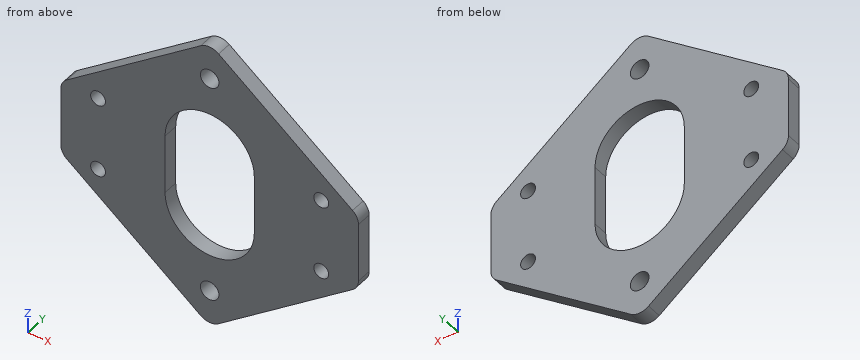
```python
from build123d import *

# Parameters (mm, degrees)
F0_R     = 12.7
F0_R_2   = 15.875
F1_DEPTH = 12.7


with BuildPart() as f1:
    # F0 (on Front) → F1 (new body, symmetric)
    with BuildSketch(Plane.XZ):
        with BuildLine():
            Line((254, -50.8), (254, 50.8))
            ThreePointArc((254, 50.8), (251.318451, 62.159225), (243.84, 71.12))
            Line((243.84, 71.12), (15.24, 242.57))
            ThreePointArc((15.24, 242.57), (0, 247.65), (-15.24, 242.57))
            Line((-15.24, 242.57), (-243.84, 71.12))
            ThreePointArc((-243.84, 71.12), (-251.318451, 62.159225), (-254, 50.8))
            Line((-254, 50.8), (-254, -50.8))
            ThreePointArc((-254, -50.8), (-251.318451, -62.159225), (-243.84, -71.12))
            Line((-243.84, -71.12), (-15.24, -242.57))
            ThreePointArc((-15.24, -242.57), (0, -247.65), (15.24, -242.57))
            Line((15.24, -242.57), (243.84, -71.12))
            ThreePointArc((243.84, -71.12), (251.318451, -62.159225), (254, -50.8))
        make_face()
        with Locations((-190.5, -63.5)):
            Circle(F0_R, mode=Mode.SUBTRACT)
        with Locations((0, -190.5)):
            Circle(F0_R_2, mode=Mode.SUBTRACT)
        with Locations((190.5, -63.5)):
            Circle(F0_R, mode=Mode.SUBTRACT)
        with Locations((-190.5, 63.5)):
            Circle(F0_R, mode=Mode.SUBTRACT)
        with BuildLine():
            ThreePointArc((-76.2, 50.8), (0, 127), (76.2, 50.8))
            Line((76.2, 50.8), (76.2, -50.8))
            ThreePointArc((76.2, -50.8), (0, -127), (-76.2, -50.8))
            Line((-76.2, -50.8), (-76.2, 50.8))
        make_face(mode=Mode.SUBTRACT)
        with Locations((190.5, 63.5)):
            Circle(F0_R, mode=Mode.SUBTRACT)
        with Locations((0, 190.5)):
            Circle(F0_R_2, mode=Mode.SUBTRACT)
    extrude(amount=F1_DEPTH, both=True)


solid = f1.part
```
The model under review builds one solid part; all positions refer to its coordinate system, in mm. Round coordinates to 2 decimals unless told otherwise and drop trailing zeros. Loops run counter-clockwise (first coordinate to the right, second up) from the corner with the lowest first, then second, coordinate; pieces in that order, holes last. Notation, with made-up numbers: (44, -31.5) - (63, -31.5) arc R21 cw to (63, -20.5) - close; hole circle Ø10 at (-31, 37). An arc over 180 degrees is marked (long way). Use a Markdown table: item, result. Add a question column.
Q1. Insertion check: pin 1 Ø15 at (x, z) = (190.5, -63.5) entering from -Y; pin 2 Ø6 at (y, z) = (-0.5, 168.5) entering from +X; pin 3 Ø2 at (x, y) = (-5.5, -9.5) entering from -Z; pin 4 Ø5 at (x, y) = (-123.5, 9) entering from +Z. Each pin has a flat end and moves straight along its axis. Give the tip position at first contact, or say it passes through.
Q2. Add section B-B (z = -181). State the section outline as (x, y) points, plus the area to 3 significant figures.
Q3. Add section D-D (x = -186). State the section outline as (y, z) points.
Q4. Add section A-A (x = 0). State the section outline as (y, z) points (3 decimals), plus the area to 3 significant figures.
Q5. Add section C-C (y = 7). State the section outline as (x, z) points (3 decimals).
Q6. For probe 1 along Z at (x, y) = (0, 6.25) (3 decimals); probe 2 along X at (y, z) = (9.5, 65); probe 3 along Z at (x, y) = (-10, 10.5), list the stretches that pass through material, from the lowest coordinate up.
Worked answers:
| question | item | result |
|---|---|---|
| 1 | pin 1 | through |
| 1 | pin 2 | x = 118 |
| 1 | pin 3 | z = -247.25 |
| 1 | pin 4 | z = 163.25 |
| 2 | outline | (-97.33, -12.7) - (-12.72, -12.7) - (-12.72, 12.7) - (-97.33, 12.7) - close; (12.72, -12.7) - (97.33, -12.7) - (97.33, 12.7) - (12.72, 12.7) - close |
| 2 | area | 4,300 mm² |
| 3 | outline | (-12.7, -114.5) - (12.7, -114.5) - (12.7, -75.38) - (-12.7, -75.38) - close; (-12.7, -51.62) - (12.7, -51.62) - (12.7, 51.62) - (-12.7, 51.62) - close; (-12.7, 75.38) - (12.7, 75.38) - (12.7, 114.5) - (-12.7, 114.5) - close |
| 4 | outline | (-12.7, -247.65) - (12.7, -247.65) - (12.7, -206.375) - (-12.7, -206.375) - close; (-12.7, -174.625) - (12.7, -174.625) - (12.7, -127) - (-12.7, -127) - close; (-12.7, 127) - (12.7, 127) - (12.7, 174.625) - (-12.7, 174.625) - close; (-12.7, 206.375) - (12.7, 206.375) - (12.7, 247.65) - (-12.7, 247.65) - close |
| 4 | area | 4,520 mm² |
| 5 | outline | (-254, -50.8) arc R25.4 ccw to (-243.84, -71.12) - (-15.24, -242.57) arc R25.4 ccw to (15.24, -242.57) - (243.84, -71.12) arc R25.4 ccw to (254, -50.8) - (254, 50.8) arc R25.4 ccw to (243.84, 71.12) - (15.24, 242.57) arc R25.4 ccw to (-15.24, 242.57) - (-243.84, 71.12) arc R25.4 ccw to (-254, 50.8) - close; hole circle Ø25.4 at (-190.5, -63.5); hole circle Ø25.4 at (-190.5, 63.5); hole (-76.2, -50.8) arc R76.2 ccw to (76.2, -50.8) - (76.2, 50.8) arc R76.2 ccw to (-76.2, 50.8) - close; hole circle Ø31.75 at (0, -190.5); hole circle Ø31.75 at (0, 190.5); hole circle Ø25.4 at (190.5, -63.5); hole circle Ø25.4 at (190.5, 63.5) |
| 6 | probe 1 | -247.65 to -206.375, -174.625 to -127, 127 to 174.625, 206.375 to 247.65 |
| 6 | probe 2 | -249.66 to -203.11, -177.89 to -74.87, 74.87 to 177.89, 203.11 to 249.66 |
| 6 | probe 3 | -245.6 to -202.83, -178.17 to -126.34, 126.34 to 178.17, 202.83 to 245.6 |
